```python
from build123d import *

# Parameters (mm, degrees)
BOSS_EXTRUDE1_DEPTH = 101.6
SKETCH2_W           = 0.8
SKETCH2_H           = 4
BOSS_EXTRUDE2_DEPTH = 12.6


with BuildPart() as part:
    # Sketch1 → Boss-Extrude1 (new body)
    with BuildSketch(Plane.XY):
        Polygon((3.1, 1.407251622), (3.1, 0.607251622), (5.5, 0.607251622), (5.5, -1.792748378), (-5.5, -1.792748378), (-5.5, 0.607251622), (-3.1, 0.607251622), (-3.1, 1.407251622), (-6.3, 1.407251622), (-6.3, -2.592748378), (6.3, -2.592748378), (6.3, 1.407251622), align=None)
    extrude(amount=BOSS_EXTRUDE1_DEPTH)

    # Sketch2 → Boss-Extrude2 (add)
    with BuildSketch(Plane.ZY.offset(6.3)):
        with Locations((-0.4, -0.592748378)):
            Rectangle(SKETCH2_W, SKETCH2_H)
    extrude(amount=-BOSS_EXTRUDE2_DEPTH)


solid = part.part
```
For this review, take the finished solid that the model builds, in its own axes (mm). A direction names the side the tool comes from. Round coordinates to 2 decimals unless told otherwise and drop trailing zeros. Write each loop counter-clockwise with the first axis right and the second up, starting at its lowest first coordinate (ties: lowest second). Pieces come first, ordered by that corner, then holes. Notation, with made-up numbers: (26, -15.5) -> (82, -15.5) arc R13 ccw to (82, 7.5) -> close; hole circle Ø9 at (36.25, 39.5). An arc over 180 degrees is marked (long way). One line per question, with ' | ' between items. Start each with the question number.
1) Add section B-B (y = -0.65). Write out the cut boundary in (x, z), and give its area (3 significant figures).
2) Wall thickness on line 1 along X through (y, z) = (-0.7, 23); line 2 along Y through (x, z) = (-3.5, 91); line 3 along X through (y, z) = (1.05, 82): over which ranges is each line inside the solid? List them lowest first.
3) Mouldability with a two-part tool opening along Y and no side actions: class faces 3 (the flat face through (0, -1, -0.8)), 4 (the flat face through (-4, 1.407, 50)), 5 (the flat face through (4, 0.607, 50)) as +Y half, -Y half, draft (parallel to the pull), parting line (faces both ways), or undercut.
4) Add section A-A (x = 4.25). Write out the cut boundary in (y, z), and give its area (3 significant figures).
5) Machinability: for faces 1 (the flat face through (-5.5, -1, 50)), 2 (the flat face through (0, -2.593, 50)), which of the approach directions +Z, -Z, +X, -X, +Y, -Y give a long, thin tool a straight path to every point of the face, cutting with its end or side? Answer none if there is none.
6) Add section C-C (z = 90.5). Write out the cut boundary in (x, y).
7) For pin 1 Ø1 at (x, y) = (-1.5, -0.5) entering from +Z, flat-tipped, find the tip position at first contact; note if it passes through.
8) Add section D-D (x = 0.5). Write out the cut boundary in (y, z), and give its area (3 significant figures).
Reported:
1) outline: (-6.3, -0.8) -> (6.3, -0.8) -> (6.3, 101.6) -> (5.5, 101.6) -> (5.5, 0) -> (-5.5, 0) -> (-5.5, 101.6) -> (-6.3, 101.6) -> close | area: 173 mm²
2) line 1: x = -6.3 to -5.5, 5.5 to 6.3 | line 2: y = -2.59 to -1.79, 0.61 to 1.41 | line 3: x = -6.3 to -3.1, 3.1 to 6.3
3) face 3: draft | face 4: +Y half | face 5: undercut
4) outline: (-2.59, -0.8) -> (1.41, -0.8) -> (1.41, 101.6) -> (0.61, 101.6) -> (0.61, 0) -> (-1.79, 0) -> (-1.79, 101.6) -> (-2.59, 101.6) -> close | area: 166 mm²
5) face 1: +Z | face 2: +Z, -Z, +X, -X, -Y
6) outline: (-6.3, -2.59) -> (6.3, -2.59) -> (6.3, 1.41) -> (3.1, 1.41) -> (3.1, 0.61) -> (5.5, 0.61) -> (5.5, -1.79) -> (-5.5, -1.79) -> (-5.5, 0.61) -> (-3.1, 0.61) -> (-3.1, 1.41) -> (-6.3, 1.41) -> close
7) pin 1: stops at z = 0
8) outline: (-2.59, -0.8) -> (1.41, -0.8) -> (1.41, 0) -> (-1.79, 0) -> (-1.79, 101.6) -> (-2.59, 101.6) -> close | area: 84.5 mm²
